Design review of the part built by this model. Coordinates are the model's own, in mm. Face numbers are marked on the shaded views. Round coordinates to 2 decimals unless told otherwise and drop trailing zeros. Order: outer loops, then holes, each group sorted by start corner. A loop starts at its lowest first (then second) coordinate and runs counter-clockwise, first axis right, second up. Notation, with made-up numbers: M -28,57.5 L -10,57.5 A26 ccw -10,79.5 Z; hole C 35.5,26 d9. An arc over 180 degrees is marked long. Use a Markdown table: item, result. Add a question column.
(1) To check wall thickness, follow probe 1 along Y at (x, z) = (-0.75, 0.95); probe 2 along Y at (x, z) = (-1.75, 0.65); probe 3 along Y at (x, z) = (-1.25, 0.7). State the ranges of each line that lie inside material, in increasing order. Write a range as from..to.
(2) Take a section at B-B (z = 0.8). Write out the cut boundary in (x, y), then the cut area to 3 significant figures.
(3) The part is to be moulded in two halves that separate along X. For the marked faces 1, 2 and 3, say which applies: released by +X, released by -X, zero draft, split by the parting line, or undercut.
(4) Take a section at D-D (y = -6.5). Write out the cut boundary in (x, z), then the cut area to 3 significant figures.
(5) Take a section at C-C (x = -1.25). Write out the cut boundary in (y, z).
(6) Take a section at A-A (y = 0.75). Write out the cut boundary in (x, z).
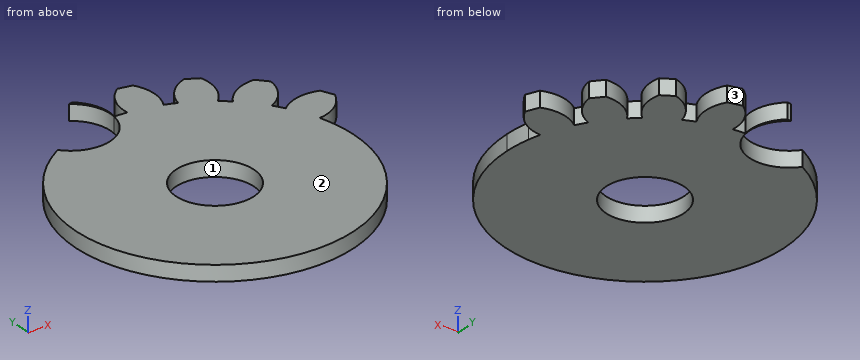
```python
from build123d import *

# Parameters (mm, degrees)
F2_R     = 2.5
F3_DEPTH = 1


# Not quite as in the source:
# - a feature of the source that left no trace in its solid (it failed there, or was rolled back) is left out


with BuildPart() as f3:
    # F2 (on Top) → F3 (new body)
    with BuildSketch(Plane.XY):
        with BuildLine():
            ThreePointArc((-0.9522931143, 11.4531284813), (-0.0520635974, 10.3538099613), (0.1218940174, 8.943613826))
            ThreePointArc((0.1218940174, 8.943613826), (0.1337416353, 8.9434445039), (0.1455890186, 8.9432594873))
            ThreePointArc((0.1455890186, 8.9432594873), (0.0799521539, 10.3250380062), (-0.6817601701, 11.4797736507))
            Line((-0.6817601701, 11.4797736507), (-0.9522931143, 11.4531284813))
        make_face()
        with BuildLine():
            ThreePointArc((-4.4173624076, 7.7775314708), (-4.4995685223, -7.7302632253), (8.9444444444, 0))
            ThreePointArc((8.9444444444, 0), (8.9053271725, 0.8356041947), (8.7883175045, 1.6638995942))
            ThreePointArc((8.7883175045, 1.6638995942), (8.7057555111, 2.0525368209), (8.6060160514, 2.4371241541))
            ThreePointArc((8.6060160514, 2.4371241541), (8.2679218833, 3.4124117792), (7.8197142384, 4.3422523705))
            ThreePointArc((7.8197142384, 4.3422523705), (7.6211518715, 4.6820007018), (7.4078378155, 5.0126864374))
            ThreePointArc((7.4078378155, 5.0126864374), (6.7776596323, 5.8366442695), (6.0563228133, 6.5820999993))
            ThreePointArc((6.0563228133, 6.5820999993), (5.761965129, 6.84126043), (5.4565297326, 7.0872681406))
            ThreePointArc((5.4565297326, 7.0872681406), (4.5991510413, 7.6714337721), (3.6798961663, 8.1523892587))
            ThreePointArc((3.6798961663, 8.1523892587), (3.3179634912, 8.306275019), (2.9496159434, 8.4441016222))
            ThreePointArc((2.9496159434, 8.4441016222), (1.9566672267, 8.7278026893), (0.937636324, 8.8951629858))
            ThreePointArc((0.937636324, 8.8951629858), (0.542146294, 8.9279988696), (0.1455890186, 8.9432594873))
            ThreePointArc((0.1455890186, 8.9432594873), (0.1337416353, 8.9434445039), (0.1218940174, 8.943613826))
            ThreePointArc((0.1218940174, 8.943613826), (-1.7655892516, 6.8729814141), (-4.4173624076, 7.7775314708))
        make_face()
        Circle(F2_R, mode=Mode.SUBTRACT)
        with BuildLine():
            ThreePointArc((7.8197142384, 4.3422523705), (8.2679218833, 3.4124117792), (8.6060160514, 2.4371241541))
            ThreePointArc((8.6060160514, 2.4371241541), (9.8961633699, 2.9277974972), (10.7564598893, 4.0072095278))
            Line((10.7564598893, 4.0072095278), (10.398401005, 4.8258001529))
            ThreePointArc((10.398401005, 4.8258001529), (9.0439881545, 4.931031832), (7.8197142384, 4.3422523705))
        make_face()
        with BuildLine():
            ThreePointArc((6.0563228133, 6.5820999993), (6.7776596323, 5.8366442695), (7.4078378155, 5.0126864374))
            ThreePointArc((7.4078378155, 5.0126864374), (8.4689810733, 5.8780879937), (8.9469442237, 7.1612466333))
            Line((8.9469442237, 7.1612466333), (8.3534515739, 7.8291263012))
            ThreePointArc((8.3534515739, 7.8291263012), (7.0378063332, 7.5133903393), (6.0563228133, 6.5820999993))
        make_face()
        with BuildLine():
            ThreePointArc((3.6798961663, 8.1523892587), (4.5991510413, 7.6714337721), (5.4565297326, 7.0872681406))
            ThreePointArc((5.4565297326, 7.0872681406), (6.194311581, 8.236914632), (6.251341492, 9.6017430828))
            Line((6.251341492, 9.6017430828), (5.4805102725, 10.0535350783))
            ThreePointArc((5.4805102725, 10.0535350783), (4.3249499065, 9.344717804), (3.6798961663, 8.1523892587))
        make_face()
        with BuildLine():
            ThreePointArc((2.0608006124, 11.2812858546), (1.1761963647, 10.2402731247), (0.937636324, 8.8951629858))
            ThreePointArc((0.937636324, 8.8951629858), (1.9566672267, 8.7278026893), (2.9496159434, 8.4441016222))
            ThreePointArc((2.9496159434, 8.4441016222), (3.3010678965, 9.7691415234), (2.9335160712, 11.08980608))
            Line((2.9335160712, 11.08980608), (2.0608006124, 11.2812858546))
        make_face()
    extrude(amount=F3_DEPTH)


solid = f3.part
```
Verdict:
| question | item | result |
|---|---|---|
| 1 | probe 1 | y = -8.91..-2.38, 2.38..7.4, 11.3..11.47 |
| 1 | probe 2 | y = -8.77..-1.79, 1.79..6.88 |
| 1 | probe 3 | y = -8.86..-2.17, 2.17..7.07 |
| 2 | outline | M -4.42,7.78 A8.94 ccw long 8.61,2.44 A2.61 ccw 10.76,4.01 L 10.4,4.83 A2.61 ccw 7.82,4.34 A8.94 ccw 7.41,5.01 A2.61 ccw 8.95,7.16 L 8.35,7.83 A2.61 ccw 6.06,6.58 A8.94 ccw 5.46,7.09 A2.61 ccw 6.25,9.6 L 5.48,10.05 A2.61 ccw 3.68,8.15 A8.94 ccw 2.95,8.44 A2.61 ccw 2.93,11.09 L 2.06,11.28 A2.61 ccw 0.94,8.9 A8.94 ccw 0.15,8.94 A2.61 ccw -0.68,11.48 L -0.95,11.45 A2.56 cw long Z; hole C 0,0 d5 |
| 2 | area | 246 mm^2 |
| 3 | face 1 | undercut |
| 3 | face 2 | zero draft |
| 3 | face 3 | released by +X |
| 4 | outline | M -6.14,0 L 6.14,0 L 6.14,1 L -6.14,1 Z |
| 4 | area | 12.3 mm^2 |
| 5 | outline | M -8.86,0 L -2.17,0 L -2.17,1 L -8.86,1 Z; M 2.17,0 L 7.07,0 L 7.07,1 L 2.17,1 Z |
| 6 | outline | M -8.91,0 L -2.38,0 L -2.38,1 L -8.91,1 Z; M 2.38,0 L 8.91,0 L 8.91,1 L 2.38,1 Z |
